Design review of the part built by this model. Coordinates are the model's own, in mm. A direction names the side the tool comes from. Give positions to 0.01 mm unless a question says otherwise; leave off trailing zeros. Loops run counter-clockwise (first coordinate to the right, second up) from the corner with the lowest first, then second, coordinate; pieces in that order, holes last. Notation, with made-up numbers: M -34,-27.75 L -19,-27.75 A4 ccw -19,-22.75 Z; hole C 23,-15 d7. An arc over 180 degrees is marked long. Use a Markdown table: item, result. Add a question column.
(1) Add section A-A, the plane x = 0. Give the boundary of the cut face in (y, z).
(2) Add section D-D, the plane z = -22. Give the boundary of the cut face in (x, y), then the cut area to 3 significant figures.
(3) Insertion check: pin 1 Ø5 at (y, z) = (7, -9.5) entering from -X; pin 2 Ø2 at (y, z) = (4, -8.5) entering from -X; pin 3 Ø6 at (x, y) = (7.5, -8) entering from +Z. Each pin has a flat end and moves straight along its axis. Give the tip position at first contact, or say it passes through.
(4) For faces 1 (the face through (-1, -6, -27.453)), 2 (the face through (24.603, 5.916, -14.057)), list the 3-axis set-ups (+Z, -Z, +X, -X, +Y, -Y) from which the entire face can be reached by the end or side of a thin tool; tool diameter is ignored.
(5) For probe 1 along Z at (x, y) = (-3.5, -0.5); probe 2 along Y at (x, z) = (34, -19.5); probe 3 along Z at (x, y) = (-30.5, 7.25), list the stretches that pass through material, from the lowest coordinate up.
(6) Add section B-B, the plane z = -2. Give the boundary of the cut face in (x, y), then the cut area to 3 significant figures.
(7) Draft analysis for pull direction Z (two halves, no side actions). For faces 3 (the face through (6.695, 5.916, 4.268)), 4 (the face through (-0.39, 5.916, 17.746)), 5 (the face through (0, 12, -15)), state which applies: pulls with the +Z half, pulls with the -Z half, needs draft (parallel to the pull), parting line crosses it, or undercut.
(8) Add section C-C, the plane y = 2.75. Give the boundary of the cut face in (x, z), then the cut area to 3 significant figures.
```python
from build123d import *

# Parameters (mm, degrees)
SKETCH1_R           = 17.75
SKETCH1_R_2         = 7.94
BOSS_EXTRUDE1_DEPTH = 12
BOSS_EXTRUDE6_DEPTH = 12
SKETCH9_W           = 80
SKETCH9_H           = 15
BOSS_EXTRUDE7_DEPTH = 12
SKETCH10_W          = 80
SKETCH10_H          = 7.5
BOSS_EXTRUDE8_DEPTH = 12


with BuildPart() as part:
    # Sketch1 → Boss-Extrude1 (new body)
    with BuildSketch(Plane(origin=(0, 0, 0), x_dir=(1, 0, 0), z_dir=(0, 1, 0))):
        with Locations(Location((0, 0, 0), (0, 0, 270))):
            Circle(SKETCH1_R)
        with Locations(Location((0, 0, 0), (0, 0, 270))):
            Circle(SKETCH1_R_2, mode=Mode.SUBTRACT)
    extrude(amount=BOSS_EXTRUDE1_DEPTH)

    # Sketch6 → Boss-Extrude6 (add)
    with BuildSketch(Plane.XZ):
        with BuildLine():
            Line((-0.456324954, -19.952681815), (-40.456324954, -19.952681815))
            ThreePointArc((-40.456324954, -19.952681815), (-25.342699441, -14.255780456), (-17.75, 0))
            ThreePointArc((-17.75, 0), (0, -17.75), (17.75, 0))
            ThreePointArc((17.75, 0), (24.769764057, -14.21114403), (39.543675046, -19.952681815))
            Line((39.543675046, -19.952681815), (-0.456324954, -19.952681815))
        make_face()
    extrude(amount=-BOSS_EXTRUDE6_DEPTH)

    # Sketch9 → Boss-Extrude7 (add)
    with BuildSketch(Plane(origin=(0, 0, 0), x_dir=(-1, 0, 0), z_dir=(0, -1, 0))):
        with Locations((0.456324954, 27.452681815)):
            Rectangle(SKETCH9_W, SKETCH9_H)
    extrude(amount=-BOSS_EXTRUDE7_DEPTH)

    # Sketch10 → Boss-Extrude8 (add)
    with BuildSketch(Plane.XZ):
        with Locations((-0.456324954, -31.202681815)):
            Rectangle(SKETCH10_W, SKETCH10_H)
    extrude(amount=BOSS_EXTRUDE8_DEPTH)


solid = part.part
```
Established:
| question | item | result |
|---|---|---|
| 1 | outline | M -12,-34.95 L 12,-34.95 L 12,-7.94 L 0,-7.94 L 0,-27.45 L -12,-27.45 Z; M 0,7.94 L 12,7.94 L 12,17.75 L 0,17.75 Z |
| 2 | outline | M -40.46,0 L 39.54,0 L 39.54,12 L -40.46,12 Z |
| 2 | area | 960 mm^2 |
| 3 | pin 1 | x = -23.11 |
| 3 | pin 2 | x = -21.24 |
| 3 | pin 3 | z = -27.45 |
| 4 | face 1 | +Z, +X, -X, -Y |
| 4 | face 2 | +Z, +X, +Y, -Y |
| 5 | probe 1 | -34.95 to -27.45 |
| 5 | probe 2 | 0 to 12 |
| 5 | probe 3 | -34.95 to -17.67 |
| 6 | outline | M -18.1,0 L -7.68,0 L -7.68,12 L -18.1,12 Z; M 7.68,0 L 18.02,0 L 18.02,12 L 7.68,12 Z |
| 6 | area | 249 mm^2 |
| 7 | face 3 | undercut |
| 7 | face 4 | pulls with the +Z half |
| 7 | face 5 | needs draft |
| 8 | outline | M -40.46,-34.95 L 39.54,-34.95 L 39.54,-19.95 A21.88 cw 17.75,0 A17.75 ccw -17.75,0 A22.9 cw -40.46,-19.95 Z; hole C 0,0 d15.88 |
| 8 | area | 2,410 mm^2 |
